The model under review builds one solid part; all positions refer to its coordinate system, in mm. A direction names the side the tool comes from. Give positions to 0.01 mm unless a question says otherwise; leave off trailing zeros. Write each loop counter-clockwise with the first axis right and the second up, starting at its lowest first coordinate (ties: lowest second). Pieces come first, ordered by that corner, then holes.
from build123d import *

# Parameters (mm, degrees)
F0_W     = 254
F0_H     = 254
F1_DEPTH = 50.8
F2_W     = 87.367308
F2_H     = 172.949922
F3_DEPTH = 127


with BuildPart() as f1:
    # F0 (on Front) → F1 (new body)
    with BuildSketch(Plane.XZ):
        with Locations((67.501718, -3.968271)):
            Rectangle(F0_W, F0_H)
    extrude(amount=F1_DEPTH)

    # F2 (on face) → F3 (join)
    with BuildSketch(Plane.XZ.offset(50.8)):
        with Locations((71.324045, 36.556768)):
            Rectangle(F2_W, F2_H)
        Polygon((-24.779992, -100.1544), (-24.779992, 123.031729), (-59.498282, 123.031729), (-59.498282, -130.968271), (194.501718, -130.968271), (194.501718, 123.031729), (166.336, 123.031729), (166.336, -100.1544), align=None)
    extrude(amount=F3_DEPTH)


solid = f1.part
1) Consider section C-C, the plane x = 91. Give the boundary of the cut face in (y, z).
2) Consider section D-D, the plane z = -72. Give the boundary of the cut face in (x, y), then the cut area to 3 significant figures.
3) The part is to be moulded in two halves that separate along Z. For faces 1 (the flat face through (-59.498, -88, -2)), 2 (the flat face through (27, -50.8, -12)), 3 (the flat face through (72, -113, -100.154)), 4 (the flat face through (66, -88, -130.968)), say which applies: +Z half, -Z half, draft (parallel to the pull), parting line (faces both ways), or undercut.
4) Consider section A-A, the plane y = -77.5. Give the boundary of the cut face in (x, z), then the cut area to 3 significant figures.
5) Consider section B-B, the plane z = -40. Give the boundary of the cut face in (x, y).
6) Tool access review of faces 5 (the flat face through (115.008, -113, 35)), 6 (the flat face through (66, 0, -2)), 7 (the flat face through (71, -113, -49.918)): name each direction out of +Z, -Z, +X, -X, +Y, -Y from which nothing blocks a thin tool from reaching the whole face with its end or side.
7) To check wall thickness, follow probe 1 along X at (y, z) = (-143.5, -5); probe 2 along X at (y, z) = (-88.5, -85.5); probe 3 along Z at (x, y) = (73, -65). State the ranges of each line that lie inside material, in increasing order.
Answer block:
1. outline: (-177.8, -130.97) - (0, -130.97) - (0, 123.03) - (-177.8, 123.03) - (-177.8, -49.92) - (-50.8, -49.92) - (-50.8, -100.15) - (-177.8, -100.15) - close
2. outline: (-59.5, -177.8) - (-24.78, -177.8) - (-24.78, -50.8) - (166.34, -50.8) - (166.34, -177.8) - (194.5, -177.8) - (194.5, 0) - (-59.5, 0) - close
2. area: 20,900 mm2
3. face 1: draft
3. face 2: undercut
3. face 3: undercut
3. face 4: -Z half
4. outline: (-59.5, -130.97) - (194.5, -130.97) - (194.5, 123.03) - (166.34, 123.03) - (166.34, -100.15) - (-24.78, -100.15) - (-24.78, 123.03) - (-59.5, 123.03) - close; (27.64, -49.92) - (115.01, -49.92) - (115.01, 123.03) - (27.64, 123.03) - close
4. area: 37,000 mm2
5. outline: (-59.5, -177.8) - (-24.78, -177.8) - (-24.78, -50.8) - (27.64, -50.8) - (27.64, -177.8) - (115.01, -177.8) - (115.01, -50.8) - (166.34, -50.8) - (166.34, -177.8) - (194.5, -177.8) - (194.5, 0) - (-59.5, 0) - close
6. face 5: +Z, -Y
6. face 6: +Z, -Z, +X, -X, +Y
6. face 7: -Y
7. probe 1: x = -59.5 to -24.78, 27.64 to 115.01, 166.34 to 194.5
7. probe 2: x = -59.5 to -24.78, 166.34 to 194.5
7. probe 3: z = -130.97 to -100.15, -49.92 to 123.03
